from build123d import *

# Parameters (mm, degrees)
SKETCH1_W           = 70
SKETCH1_H           = 15
BOSS_EXTRUDE1_DEPTH = 2
BOSS_EXTRUDE2_START = -2
SKETCH2_R           = 7.5
BOSS_EXTRUDE2_DEPTH = 2
SKETCH3_R           = 3.2
SKETCH3_R_2         = 2.4
BOSS_EXTRUDE5_DEPTH = 20
SKETCH10_R          = 2.4
CUT_EXTRUDE1_DEPTH  = 16
SKETCH11_R          = 3.2
SKETCH11_R_2        = 2.199750497
BOSS_EXTRUDE6_DEPTH = 22
SKETCH12_R          = 2.2
SKETCH12_R_2        = 2
BOSS_EXTRUDE8_DEPTH = 22
SKETCH13_R          = 2.2
CUT_EXTRUDE2_DEPTH  = 4
SKETCH14_R          = 2.5
SKETCH14_R_2        = 2
CUT_EXTRUDE4_DEPTH  = 17


with BuildPart() as part:
    # Sketch1 → Boss-Extrude1 (new body)
    with BuildSketch(Plane(origin=(0, 0, 0), x_dir=(1, 0, 0), z_dir=(0, 1, 0))):
        with Locations((35, 7.5)):
            Rectangle(SKETCH1_W, SKETCH1_H)
    extrude(amount=BOSS_EXTRUDE1_DEPTH)

    # Sketch2 → Boss-Extrude2 (add)
    with BuildSketch(Plane(origin=(0, 2, 0), x_dir=(1, 0, 0), z_dir=(0, 1, 0)).offset(BOSS_EXTRUDE2_START)):
        with Locations((0, 7.5)):
            Circle(SKETCH2_R)
    extrude(amount=BOSS_EXTRUDE2_DEPTH)

    # Sketch3 → Boss-Extrude5 (add)
    with BuildSketch(Plane(origin=(0, 2, 0), x_dir=(1, 0, 0), z_dir=(0, 1, 0))):
        with Locations((0, 7.5)):
            Circle(SKETCH3_R)
        with Locations((0, 7.5)):
            Circle(SKETCH3_R_2, mode=Mode.SUBTRACT)
    extrude(amount=BOSS_EXTRUDE5_DEPTH)

    # Sketch10 → Cut-Extrude1 (cut)
    with BuildSketch(Plane(origin=(0, 2, 0), x_dir=(1, 0, 0), z_dir=(0, 1, 0))):
        with Locations((0, 7.5)):
            Circle(SKETCH10_R)
    extrude(amount=-CUT_EXTRUDE1_DEPTH, mode=Mode.SUBTRACT)

    # Sketch11 → Boss-Extrude6 (add)
    with BuildSketch(Plane(origin=(0, 22, 0), x_dir=(1, 0, 0), z_dir=(0, 1, 0))):
        with Locations((0, 7.5)):
            Circle(SKETCH11_R)
        with Locations((0, 7.5)):
            Circle(SKETCH11_R_2, mode=Mode.SUBTRACT)
    extrude(amount=-BOSS_EXTRUDE6_DEPTH)

    # Sketch12 → Boss-Extrude8 (add)
    with BuildSketch(Plane(origin=(0, 22, 0), x_dir=(1, 0, 0), z_dir=(0, 1, 0))):
        with Locations((0, 7.5)):
            Circle(SKETCH12_R)
        with Locations((0, 7.5)):
            Circle(SKETCH12_R_2, mode=Mode.SUBTRACT)
    extrude(amount=-BOSS_EXTRUDE8_DEPTH)

    # Sketch13 → Cut-Extrude2 (cut)
    with BuildSketch(Plane(origin=(0, 22, 0), x_dir=(1, 0, 0), z_dir=(0, 1, 0))):
        with Locations((0, 7.5)):
            Circle(SKETCH13_R)
    extrude(amount=-CUT_EXTRUDE2_DEPTH, mode=Mode.SUBTRACT)

    # Sketch14 → Cut-Extrude4 (cut)
    with BuildSketch(Plane.XZ):
        with Locations((0, -7.5)):
            Circle(SKETCH14_R)
        with Locations((0, -7.5)):
            Circle(SKETCH14_R_2, mode=Mode.SUBTRACT)
    extrude(amount=-CUT_EXTRUDE4_DEPTH, mode=Mode.SUBTRACT)


solid = part.part
Read the model definition and answer for the solid it produces. Units are mm, in the model's axes. A direction names the side the tool comes from. Coordinates: 2 decimals unless noted, no trailing zeros. Write each loop counter-clockwise with the first axis right and the second up, starting at its lowest first coordinate (ties: lowest second). Pieces come first, ordered by that corner, then holes. Notation, with made-up numbers: (76.5, 12) -> (134.5, 12) arc R20 ccw to (134.5, 25) -> close; hole circle Ø1 at (1, -4). An arc over 180 degrees is marked (long way). Return JSON: item names as keys, results as strings.
(1) The part is cut by section D-D on z = -2.5. Give the vertices of the cut face in (x, y), then the cut area to 3 significant figures.
Answers below:
{"outline": "(-5.59, 0) -> (70, 0) -> (70, 2) -> (-5.59, 2) -> close", "area": "151 mm^2"}
(2) The part is cut by section B-B on y = 5.25. Give the vertices of the cut face in (x, z).
Answers below:
{"outline": "circle Ø6.4 at (0, -7.5); hole circle Ø5 at (0, -7.5)"}
(3) Consider line 1 along Z through (x, y) = (0, 12.5); line 2 along Z through (x, y) = (0, 17.8); line 3 along X through (y, z) = (17.4, -7.5). Determine where each line is inside the solid, lowest interval first. Write a range as from..to.
Answers below:
{"line 1": "-10.7..-10, -5..-4.3", "line 2": "-10.7..-9.5, -5.5..-4.3", "line 3": "-3.2..-2, 2..3.2"}
(4) The part is cut by section A-A on z = -7.5. Give the vertices of the cut face in (x, y), then the cut area to 3 significant figures.
Answers below:
{"outline": "(-7.5, 0) -> (-2.5, 0) -> (-2.5, 17) -> (-2, 17) -> (-2, 18) -> (-2.2, 18) -> (-2.2, 22) -> (-3.2, 22) -> (-3.2, 2) -> (-7.5, 2) -> close; (2, 17) -> (2.5, 17) -> (2.5, 0) -> (70, 0) -> (70, 2) -> (3.2, 2) -> (3.2, 22) -> (2.2, 22) -> (2.2, 18) -> (2, 18) -> close", "area": "176 mm^2"}
(5) The part is cut by section C-C on x = 33.5. Give the vertices of the cut face in (y, z), then the cut area to 3 significant figures.
Answers below:
{"outline": "(0, -15) -> (2, -15) -> (2, 0) -> (0, 0) -> close", "area": "30.0 mm^2"}
(6) Each of these flat-tipped pins is pushed along its axis until it touches: P1, Ø7.5, axis at x = 35, z = -8.5, coming from the +Y side; P2, Ø7, axis at x = 0, z = -7.5, coming from the +Y side; P3, Ø4, axis at y = 17, z = -7, coming from the +X side; P4, Ø1.3, axis at x = 0, z = -7.5, coming from the +Y side. Where does it stop, or does it pass through?
Answers below:
{"P1": "y = 2", "P2": "y = 22", "P3": "x = 3.2", "P4": "through"}
(7) Which of the six approach directions +Z, -Z, +X, -X, +Y, -Y give full straight-line access (tool end or side, diameter ignored) to faces 1 (the cylindrical face through (-0.54, 8.38, -9.94)), 2 (the cylindrical face through (1.183, 20.028, -9.355)), 3 (the flat face through (35, 1, 0))?
Answers below:
{"face 1": "-Y", "face 2": "+Y", "face 3": "+Z, +X, -X, +Y, -Y"}
(8) For a pull along Z with two mould halves and no side action, classify faces 4 (the flat face through (35, 1, -15)), 5 (the flat face through (31, 0, -8)), 6 (the cylindrical face through (-0.26, 17.507, -9.483)) as pulls with the +Z half, pulls with the -Z half, needs draft (parallel to the pull), parting line crosses it, or undercut.
Answers below:
{"face 4": "pulls with the -Z half", "face 5": "needs draft", "face 6": "undercut"}
